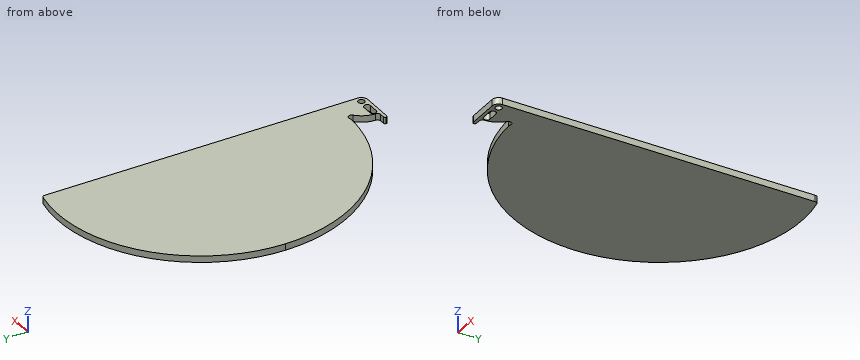
```python
from build123d import *
from OCP.BRepFilletAPI import BRepFilletAPI_MakeFillet

# Parameters (mm, degrees)
SKETCH2_R           = 0.5
BOSS_EXTRUDE1_DEPTH = 0.5
FILLET1_R           = 0.5
FILLET1_R_2         = 0.25


with BuildPart() as part:
    # Sketch2 → Boss-Extrude1 (new, symmetric)
    with BuildSketch(Plane.XY):
        with BuildLine():
            Line((0, -1.5), (0, 47.174281802))
            ThreePointArc((0, 47.174281802), (-18.674791912, 42.983685528), (-26.999996608, 25.75))
            ThreePointArc((-26.999996608, 25.75), (-20.318377061, 9.259170115), (-4.081325301, 1.982518397))
            ThreePointArc((-4.081325301, 1.982518397), (-3.375535656, 1.939379355), (-3.418674699, 1.23358971))
            ThreePointArc((-3.418674699, 1.23358971), (-4.423027454, -0.232962886), (-4.615591238, -2))
            Line((-4.615591238, -2), (-6.115591238, -2))
            Line((-6.115591238, -2), (-6.115591238, -2.5))
            Line((-6.115591238, -2.5), (-1, -2.5))
            ThreePointArc((-1, -2.5), (-0.292893219, -2.207106781), (0, -1.5))
        make_face()
        with Locations((-1, -1.5)):
            Circle(SKETCH2_R, mode=Mode.SUBTRACT)
        with BuildLine():
            Line((-4, -1), (-2.5, -1))
            ThreePointArc((-2.5, -1), (-2, -1.5), (-2.5, -2))
            Line((-2.5, -2), (-4, -2))
            ThreePointArc((-4, -2), (-4.5, -1.5), (-4, -1))
        make_face(mode=Mode.SUBTRACT)
    extrude(amount=BOSS_EXTRUDE1_DEPTH, both=True)

    # Fillet1
    fillet1_edges_1 = [part.edges().sort_by_distance(p)[0] for p in [
        (-4.081325301, 1.982518397, 0),
        (-4.615591238, -2, 0),
        (0, 47.174281802, 0),
    ]]
    fillet1_edges_2 = [part.edges().sort_by_distance(p)[0] for p in [
        (-6.115591238, -2.5, 0),
        (-6.115591238, -2, 0),
    ]]
    fillet1 = BRepFilletAPI_MakeFillet(part.part.solid().wrapped)
    for e in fillet1_edges_1:
        fillet1.Add(FILLET1_R - 0.0001, e.wrapped)
    for e in fillet1_edges_2:
        fillet1.Add(FILLET1_R_2 - 0.0001, e.wrapped)
    add(Compound.cast(fillet1.Shape()), mode=Mode.REPLACE)  # a hair under: the kernel refuses the full size


solid = part.part
```
Check sheet for the modelled part. Datum: model origin and axes. Units: mm. Round coordinates to 2 decimals unless told otherwise and drop trailing zeros. Order: outer loops, then holes, each group sorted by start corner. A loop starts at its lowest first (then second) coordinate and runs counter-clockwise, first axis right, second up. Notation, with made-up numbers: (26, 8.25) -> (49, 8.25) arc R22 cw to (49, 19.25) -> close; hole circle Ø7 at (-6.5, 72.5). An arc over 180 degrees is marked (long way). One line per item, written item: value. Start each with the question number.
Q1. Cross-section at A-A (z = -0.15). Give the number of separate pieces and of enclosed holes in the cut face, and give its area (3 significant figures).
Q2. Thickness scan on line 1 (Y direction, x = -1, z = 0.3); line 2 (Y direction, x = -2.5, z = 0.2); line 3 (X direction, y = 40, z = 0.3). Record the ranges inside material, lowest first.
Q3. Cross-section at C-C (y = 33). Record the boundary of the cut face in (x, z).
Q4. Cross-section at B-B (x = -9.25). Record the boundary of the cut face in (y, z).
Completed:
1. separate pieces: 1
1. enclosed holes: 2
1. area: 1,030 mm²
2. line 1: y = -2.5 to -2, -1 to 47.38
2. line 2: y = -2.5 to -2, -1 to 47.61
2. line 3: x = -21.76 to 0
3. outline: (-25.77, -0.5) -> (0, -0.5) -> (0, 0.5) -> (-25.77, 0.5) -> close
4. outline: (2.76, -0.5) -> (47.34, -0.5) -> (47.34, 0.5) -> (2.76, 0.5) -> close
